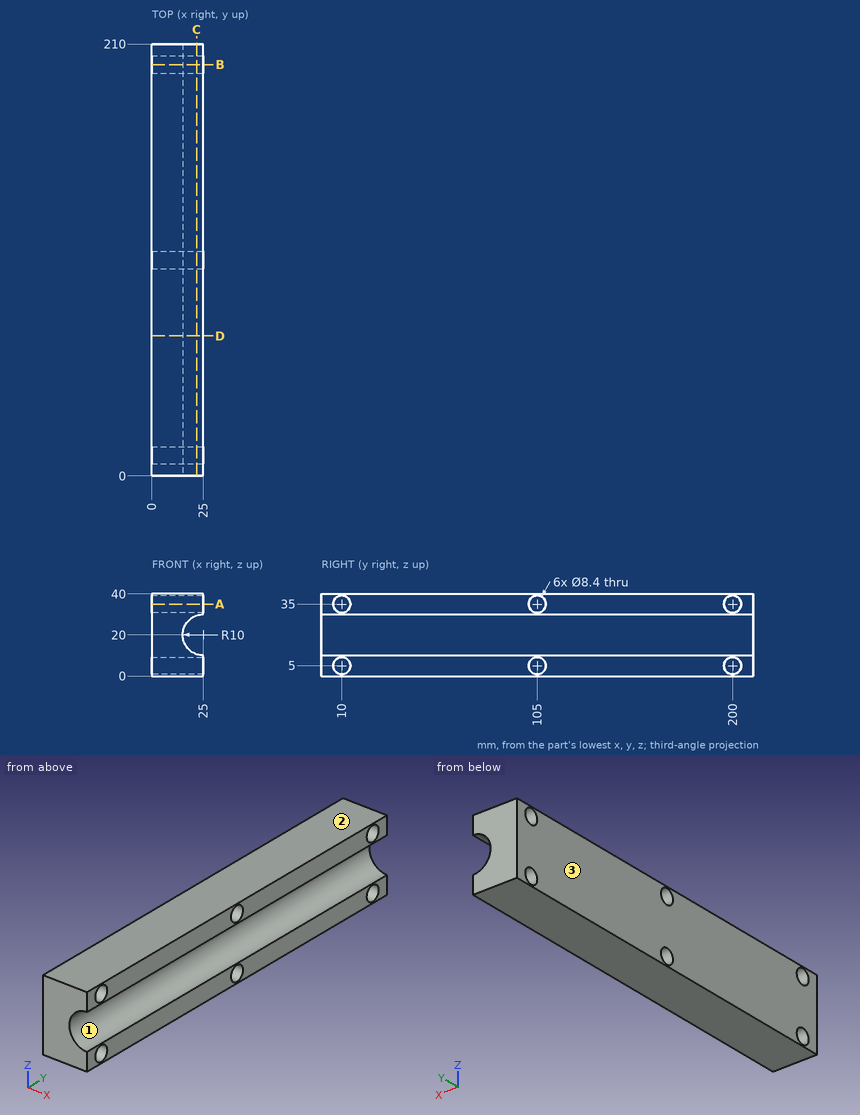
For this review, use the dimensioned drawing (mm, ordinates from the lowest corner) and the shaded views. Coordinates: 2 decimals unless noted, no trailing zeros. Write each loop counter-clockwise with the first axis right and the second up, starting at its lowest first coordinate (ties: lowest second). Pieces come first, ordered by that corner, then holes. Notation, with made-up numbers: (19, -1.75) - (32, -1.75) arc R31 cw to (32, 37.25) - close; hole circle Ø9 at (59.25, -38). An arc over 180 degrees is marked (long way). Answer as a JSON object with one key per item and string values. Group by question number.
1. Mouldability with a two-part tool opening along Z and no side actions: class the marked faces 1, 2 and 3 as pulls with the +Z half, pulls with the -Z half, needs draft (parallel to the pull), parting line crosses it, or undercut.
2. Clearance check with a flat-ended pin moving along its axis: pin 1 Ø7.5 at (y, z) = (10, 35) entering from -X (3 decimals). State where the tip first meets the part, or that it passes through.
3. Add section C-C (x = 21.75). Give the boundary of the cut face in (y, z).
4. Add section D-D (y = 68). Give the boundary of the cut face in (x, z).
5. Add section B-B (y = 200). Give the boundary of the cut face in (x, z).
6. To check wall thickness, follow probe 1 along Y at (x, z) = (9.5, 35); probe 2 along Z at (x, y) = (12.75, 105); probe 3 along Y at (x, z) = (12.25, 7.5). State the ranges of each line that lie inside material, in increasing order.
7. Add section A-A (z = 35). Give the boundary of the cut face in (x, y), plus the area to 3 significant figures.
Findings:
{
 "1": {"face 1": "undercut", "face 2": "pulls with the +Z half", "face 3": "needs draft"},
 "2": {"pin 1": "through"},
 "3": {"outline": "(0, 0) - (210, 0) - (210, 10.54) - (0, 10.54) - close; (0, 29.46) - (210, 29.46) - (210, 40) - (0, 40) - close; hole circle Ø8.4 at (10, 5); hole circle Ø8.4 at (10, 35); hole circle Ø8.4 at (105, 5); hole circle Ø8.4 at (105, 35); hole circle Ø8.4 at (200, 5); hole circle Ø8.4 at (200, 35)"},
 "4": {"outline": "(0, 0) - (25, 0) - (25, 10) arc R10 cw to (25, 30) - (25, 40) - (0, 40) - close"},
 "5": {"outline": "(0, 0) - (25, 0) - (25, 0.8) - (0, 0.8) - close; (0, 9.2) - (25, 9.2) - (25, 10) arc R10 cw to (25, 30) - (25, 30.8) - (0, 30.8) - close; (0, 39.2) - (25, 39.2) - (25, 40) - (0, 40) - close"},
 "6": {"probe 1": "0 to 5.8, 14.2 to 100.8, 109.2 to 195.8, 204.2 to 210", "probe 2": "0 to 0.8, 9.2 to 30.8, 39.2 to 40", "probe 3": "0 to 6.63, 13.37 to 101.63, 108.37 to 196.63, 203.37 to 210"},
 "7": {"outline": "(0, 0) - (25, 0) - (25, 5.8) - (0, 5.8) - close; (0, 14.2) - (25, 14.2) - (25, 100.8) - (0, 100.8) - close; (0, 109.2) - (25, 109.2) - (25, 195.8) - (0, 195.8) - close; (0, 204.2) - (25, 204.2) - (25, 210) - (0, 210) - close", "area": "4,620 mm²"}
}
